Part model, mm, in its own coordinate system. A direction names the side the tool comes from. Coordinates: 2 decimals unless noted, no trailing zeros. Order: outer loops, then holes, each group sorted by start corner. A loop starts at its lowest first (then second) coordinate and runs counter-clockwise, first axis right, second up.
from build123d import *

# Parameters (mm, degrees)
SKETCH_1_W           = 99.974800609
SKETCH_1_H           = 51.97470409
EXTRUDE_1_DEPTH      = 8.6
SKETCH_2_W           = 95.974800609
SKETCH_2_H           = 47.97470409
CUT_EXTRUDE_1_DEPTH  = 4
SKETCH_3_W           = 2
SKETCH_3_H           = 10
SKETCH_3_H_2         = 9.97470409
CUT_EXTRUDE_2_DEPTH  = 3.35
SKETCH_4_R           = 1.1
SKETCH_4_W           = 38.392586289
SKETCH_4_H           = 7.4
SKETCH_4_W_2         = 5.95
SKETCH_4_H_2         = 5.95
CUT_EXTRUDE_3_DEPTH  = 1437.448457956
FILLET_1_R           = 3
FILLET_3_R           = 2
SKETCH_12_W          = 9.000025401
SKETCH_12_H          = 9.0000508
EXTRUDE_3_DEPTH      = 2.7
SKETCH_13_W          = 16.992125984
SKETCH_13_H          = 17.047314393
EXTRUDE_4_DEPTH      = 1.9
SKETCH_7_W           = 53.6
SKETCH_7_H           = 10.97470409
CUT_EXTRUDE_14_DEPTH = 4
FILLET_7_R           = 2
FILLET_8_R           = 1
SKETCH_14_W          = 2.323736835
SKETCH_14_H          = 6.8
CUT_EXTRUDE_15_DEPTH = 2
SKETCH_15_W          = 4.3
SKETCH_15_H          = 51.97470409
CUT_EXTRUDE_16_DEPTH = 1490.156636733


with BuildPart() as part:
    # 草图1 → 凸台-拉伸1 (new body)
    with BuildSketch(Plane.XY.offset(1046.483288979)):
        with Locations((934.375963031, 1020.144466268)):
            Rectangle(SKETCH_1_W, SKETCH_1_H)
    extrude(amount=EXTRUDE_1_DEPTH)

    # 草图2 → 切除-拉伸1 (cut)
    with BuildSketch(Plane(origin=(0, 0, 1046.483288979), x_dir=(-1, 0, 0), z_dir=(0, 0, -1))):
        with Locations((-934.375963031, 1020.144466268)):
            Rectangle(SKETCH_2_W, SKETCH_2_H)
    extrude(amount=-CUT_EXTRUDE_1_DEPTH, mode=Mode.SUBTRACT)

    # 草图3 → 切除-拉伸2 (cut)
    with BuildSketch(Plane(origin=(0, 0, 1046.483288979), x_dir=(-1, 0, 0), z_dir=(0, 0, -1))):
        with Locations((-885.388562726, 1034.131818313)):
            Rectangle(SKETCH_3_W, SKETCH_3_H)
        with Locations((-885.388562726, 1020.144466268)):
            Rectangle(SKETCH_3_W, SKETCH_3_H_2)
        with Locations((-885.388562726, 1006.157114223)):
            Rectangle(SKETCH_3_W, SKETCH_3_H)
    extrude(amount=-CUT_EXTRUDE_2_DEPTH, mode=Mode.SUBTRACT)

    # 草图4 → 切除-拉伸3 (cut, through all)
    with BuildSketch(Plane(origin=(0, 0, 1050.483288979), x_dir=(-1, 0, 0), z_dir=(0, 0, -1))):
        with Locations((-920.388562726, 1041.631818313)):
            Circle(SKETCH_4_R)
        with Locations((-920.388562726, 998.657114223)):
            Circle(SKETCH_4_R)
        with Locations((-972.363363335, 998.657114223)):
            Circle(SKETCH_4_R)
        with Locations((-972.363363335, 1041.631818313)):
            Circle(SKETCH_4_R)
        with Locations((-949.933821712, 1001.144429438)):
            Rectangle(SKETCH_4_W, SKETCH_4_H)
        with Locations((-977.376048121, 1035.144495478)):
            Rectangle(SKETCH_4_W_2, SKETCH_4_H_2)
    extrude(amount=-CUT_EXTRUDE_3_DEPTH, mode=Mode.SUBTRACT)

    # 圆角1
    fillet_1_edges = [part.edges().sort_by_distance(p)[0] for p in [
        (884.388562726, 1046.131818313, 1050.783288979),
        (984.363363335, 1046.131818313, 1050.783288979),
        (984.363363335, 994.157114223, 1050.783288979),
        (884.388562726, 994.157114223, 1050.783288979),
    ]]
    fillet(fillet_1_edges, radius=FILLET_1_R)

    # 圆角3
    fillet_3_edges = [part.edges().sort_by_distance(p)[0] for p in [
        (980.351048121, 1032.169495478, 1052.783288979),
        (980.351048121, 1038.119495478, 1052.783288979),
        (974.401048121, 1038.119495478, 1052.783288979),
        (974.401048121, 1032.169495478, 1052.783288979),
    ]]
    fillet(fillet_3_edges, radius=FILLET_3_R)

    # 草图12 → 凸台-拉伸3 (add)
    with BuildSketch(Plane(origin=(0, 0, 1050.483288979), x_dir=(-1, 0, 0), z_dir=(0, 0, -1))):
        with Locations((-955.369926709, 1022.842410134)):
            Rectangle(SKETCH_12_W, SKETCH_12_H)
    extrude(amount=EXTRUDE_3_DEPTH)

    # 草图13 → 凸台-拉伸4 (add)
    with BuildSketch(Plane(origin=(0, 0, 1050.483288979), x_dir=(-1, 0, 0), z_dir=(0, 0, -1))):
        with Locations((-935.979052947, 1018.778239857)):
            Rectangle(SKETCH_13_W, SKETCH_13_H)
    extrude(amount=EXTRUDE_4_DEPTH)

    # 草图7 → 切除-拉伸14 (cut)
    with BuildSketch(Plane.XY.offset(1055.083288979)):
        Polygon((885.888562726, 1019.831818313), (982.863363335, 1019.831818313), (982.863363335, 1008.131818313), (927.763363335, 1008.131818313), (927.763363335, 1006.631818313), (927.763363335, 995.657114223), (885.888562726, 995.657114223), align=None)
        Polygon((934.163363335, 1044.631818313), (934.163363335, 1033.131818313), (935.663363335, 1033.131818313), (935.663363335, 1044.631818313), (982.863363335, 1044.631818313), (982.863363335, 1021.331818313), (963.463363335, 1021.331818313), (963.463363335, 1032.731818313), (943.963363335, 1032.731818313), (943.963363335, 1031.231818313), (961.963363335, 1031.231818313), (961.963363335, 1021.331818313), (927.563363335, 1021.331818313), (927.563363335, 1032.811818313), (904.363363335, 1032.811818313), (904.363363335, 1044.631818313), align=None)
        with Locations((956.063363335, 1001.144466268)):
            Rectangle(SKETCH_7_W, SKETCH_7_H)
        Polygon((926.063363335, 1021.331818313), (926.063363335, 1031.311818313), (902.863363335, 1031.311818313), (902.863363335, 1044.631818313), (885.888562726, 1044.631818313), (885.888562726, 1021.331818313), align=None)
    extrude(amount=-CUT_EXTRUDE_14_DEPTH, mode=Mode.SUBTRACT)

    # 圆角7
    fillet_7_edges = [part.edges().sort_by_distance(p)[0] for p in [
        (982.363363335, 996.157114223, 1048.483288979),
        (982.363363335, 1044.131818313, 1048.483288979),
        (886.388562726, 1044.131818313, 1048.483288979),
        (886.388562726, 996.157114223, 1048.483288979),
        (982.863363335, 995.657114223, 1053.083288979),
        (929.263363335, 995.657114223, 1053.083288979),
        (929.263363335, 1006.631818313, 1053.083288979),
        (982.863363335, 1006.631818313, 1053.083288979),
        (961.963363335, 1021.331818313, 1053.083288979),
        (927.563363335, 1021.331818313, 1053.083288979),
        (927.563363335, 1032.811818313, 1053.083288979),
        (904.363363335, 1032.811818313, 1053.083288979),
        (904.363363335, 1044.631818313, 1053.083288979),
        (934.163363335, 1044.631818313, 1053.083288979),
        (935.663363335, 1044.631818313, 1053.083288979),
        (982.863363335, 1044.631818313, 1053.083288979),
        (982.863363335, 1021.331818313, 1053.083288979),
        (963.463363335, 1021.331818313, 1053.083288979),
        (963.463363335, 1032.731818313, 1053.083288979),
        (961.963363335, 1031.231818313, 1053.083288979),
        (885.888562726, 1021.331818313, 1053.083288979),
        (885.888562726, 1044.631818313, 1053.083288979),
        (902.863363335, 1044.631818313, 1053.083288979),
        (902.863363335, 1031.311818313, 1053.083288979),
        (926.063363335, 1031.311818313, 1053.083288979),
        (926.063363335, 1021.331818313, 1053.083288979),
        (927.763363335, 995.657114223, 1053.083288979),
        (885.888562726, 995.657114223, 1053.083288979),
        (885.888562726, 1019.831818313, 1053.083288979),
        (982.863363335, 1019.831818313, 1053.083288979),
        (982.863363335, 1008.131818313, 1053.083288979),
        (927.763363335, 1008.131818313, 1053.083288979),
    ]]
    fillet(fillet_7_edges, radius=FILLET_7_R)

    # 圆角8
    fillet_8_edges = [part.edges().sort_by_distance(p)[0] for p in [
        (930.737528567, 997.444429438, 1050.783288979),
        (969.130114856, 997.444429438, 1050.783288979),
        (930.737528567, 1004.844429438, 1050.783288979),
        (969.130114856, 1004.844429438, 1050.783288979),
    ]]
    fillet(fillet_8_edges, radius=FILLET_8_R)

    # 草图14 → 切除-拉伸15 (cut)
    with BuildSketch(Plane.XY.offset(1055.083288979)):
        with Locations((983.201494917, 1013.231818313)):
            Rectangle(SKETCH_14_W, SKETCH_14_H)
    extrude(amount=-CUT_EXTRUDE_15_DEPTH, mode=Mode.SUBTRACT)

    # 草图15 → 切除-拉伸16 (cut, through all)
    with BuildSketch(Plane(origin=(984.363363335, 0, 0), x_dir=(0, 0, -1), z_dir=(1, 0, 0))):
        with Locations((-1048.633288979, 1020.144466268)):
            Rectangle(SKETCH_15_W, SKETCH_15_H)
    extrude(amount=-CUT_EXTRUDE_16_DEPTH, mode=Mode.SUBTRACT)


solid = part.part
Q1. Cut at D-D on x = 909. Write the cut outline in (y, z).
Results list:
outline: (994.16, 1050.78) - (1046.13, 1050.78) - (1046.13, 1055.08) - (1044.63, 1055.08) - (1044.63, 1051.08) - (1032.81, 1051.08) - (1032.81, 1055.08) - (1031.31, 1055.08) - (1031.31, 1051.08) - (1021.33, 1051.08) - (1021.33, 1055.08) - (1019.83, 1055.08) - (1019.83, 1051.08) - (995.66, 1051.08) - (995.66, 1055.08) - (994.16, 1055.08) - close
Q2. Cut at C-C on z = 1054.25. Count the separate pieces of the cut face and the enclosed holes in it, and give its area (3 significant figures).
Results list:
separate pieces: 1
enclosed holes: 3
area: 822 mm2
Q3. Cut at A-A on x = 946. Write the cut outline in (y, z), and give its area (3 significant figures).
Results list:
outline: (994.16, 1050.78) - (997.44, 1050.78) - (997.44, 1051.08) - (995.66, 1051.08) - (995.66, 1055.08) - (994.16, 1055.08) - close; (1004.84, 1050.78) - (1046.13, 1050.78) - (1046.13, 1055.08) - (1044.63, 1055.08) - (1044.63, 1051.08) - (1032.73, 1051.08) - (1032.73, 1055.08) - (1031.23, 1055.08) - (1031.23, 1051.08) - (1021.33, 1051.08) - (1021.33, 1055.08) - (1019.83, 1055.08) - (1019.83, 1051.08) - (1008.13, 1051.08) - (1008.13, 1055.08) - (1006.63, 1055.08) - (1006.63, 1051.08) - (1004.84, 1051.08) - close
area: 43.4 mm2
Q4. Mould opens along X. For faces 3 (the face through (919, 1044.632, 1053)), 4 (the face through (934, 1046.132, 1053)), 5 (the face through (983.46, 995.01, 1052.96)) say: pulls with the +X half, pulls with the -X half, needs draft (parallel to the pull), parting line crosses it, or undercut.
Results list:
face 3: undercut
face 4: needs draft
face 5: pulls with the +X half
Q5. Cut at B-B on y = 1015. Write the cut outline in (x, z).
Results list:
outline: (884.39, 1050.78) - (984.36, 1050.78) - (984.36, 1053.08) - (982.86, 1053.08) - (982.86, 1051.08) - (885.89, 1051.08) - (885.89, 1055.08) - (884.39, 1055.08) - close
Q6. Pin check, flat tip, straight feed: pin 1 Ø1.5 at (x, y) = (896, 1027) entering from +Z. Stop position of the tip, or through.
Results list:
pin 1: stops at z = 1051.08
Q7. Which spindle directions (+Z, -Z, +X, -X, +Y, -Y) get a long thin tool onto all of the face, cutting with end or side? Do faces 1 (the face through (983.46, 1045.28, 1052.96)), 2 (the face through (886.46, 1021.93, 1053.06)). Say none if no direction does.
Results list:
face 1: +Z, -Z, +X, +Y
face 2: +Z
Q8. Wall check: line 1 along Y through (x, z) = (966, 1051.9); line 2 along Y through (x, z) = (945.5, 1053.6); line 3 along Y through (x, z) = (899.5, 1053.9). Give the ranges that are in metal, low to high.
Results list:
line 1: y = 994.16 to 995.66, 1006.63 to 1008.13, 1019.83 to 1021.33, 1044.63 to 1046.13
line 2: y = 994.16 to 995.66, 1006.63 to 1008.13, 1019.83 to 1021.33, 1031.23 to 1032.73, 1044.63 to 1046.13
line 3: y = 994.16 to 995.66, 1019.83 to 1021.33, 1044.63 to 1046.13
